Verification items for the finished model (mm, model axes). A direction names the side the tool comes from. Round coordinates to 2 decimals unless told otherwise and drop trailing zeros. Loops run counter-clockwise (first coordinate to the right, second up) from the corner with the lowest first, then second, coordinate; pieces in that order, holes last. Notation, with made-up numbers: M 77.25,24.5 L 123.25,24.5 A13 cw 123.25,47.5 Z; hole C 32.25,19 d2. An arc over 180 degrees is marked long. One line per item, written item: value.
from build123d import *

# Parameters (mm, degrees)
SKETCH_1_W          = 20
SKETCH_1_H          = 20
EXTRUDE_1_DEPTH     = 490
SKETCH_2_W          = 14
SKETCH_2_H          = 14
CUT_EXTRUDE_1_DEPTH = 491
SKETCH_3_R          = 1.5
CUT_EXTRUDE_2_DEPTH = 80
SKETCH_4_R          = 1.55
CUT_EXTRUDE_3_DEPTH = 27


with BuildPart() as part:
    # 草图1 → 凸台-拉伸1 (new body)
    with BuildSketch(Plane.XY):
        with Locations((0.666666667, 1.006147649)):
            Rectangle(SKETCH_1_W, SKETCH_1_H)
    extrude(amount=EXTRUDE_1_DEPTH)

    # 草图2 → 切除-拉伸1 (cut, through all)
    with BuildSketch(Plane(origin=(0, 0, 0), x_dir=(-1, 0, 0), z_dir=(0, 0, -1))):
        with Locations((-0.666666667, 1.006147649)):
            Rectangle(SKETCH_2_W, SKETCH_2_H)
    extrude(amount=-CUT_EXTRUDE_1_DEPTH, mode=Mode.SUBTRACT)

    # 草图3 → 切除-拉伸2 (cut)
    with BuildSketch(Plane(origin=(10.666666667, 0, 0), x_dir=(0, 0, -1), z_dir=(1, 0, 0))):
        with Locations((-477, 1.006147649)):
            Circle(SKETCH_3_R)
        with Locations((-457, 1.006147649)):
            Circle(SKETCH_3_R)
        with Locations((-437, 1.006147649)):
            Circle(SKETCH_3_R)
    extrude(amount=-CUT_EXTRUDE_2_DEPTH, mode=Mode.SUBTRACT)

    # 草图4 → 切除-拉伸3 (cut)
    with BuildSketch(Plane.ZY.offset(9.333333333)):
        with Locations((13, 1.006147649)):
            Circle(SKETCH_4_R)
        with Locations((33, 1.006147649)):
            Circle(SKETCH_4_R)
        with Locations((53, 1.006147649)):
            Circle(SKETCH_4_R)
    extrude(amount=-CUT_EXTRUDE_3_DEPTH, mode=Mode.SUBTRACT)


solid = part.part
(1) Depth check by flat-ended pin: pin 1 Ø2.5 at (y, z) = (1.01, 457) entering from -X. Enter the tip coordinate at first touch or a pass-through.
Completed:
pin 1: passes through
(2) Sectioned sample at A-A on z = 424.5. Enter the section's corners in (x, y), and give its area (3 significant figures).
Completed:
outline: M -9.33,-8.99 L 10.67,-8.99 L 10.67,11.01 L -9.33,11.01 Z; hole M -6.33,-5.99 L 7.67,-5.99 L 7.67,8.01 L -6.33,8.01 Z
area: 204 mm^2
(3) Thickness scan on L1, parallel to X at y = 7.5, z = 412; L2, parallel to Y at x = 0.75, z = 87; L3, parallel to Y at x = 9.65, z = 13. Record the ranges inside material, lowest first. Write a range as from..to.
Completed:
L1: x = -9.33..-6.33, 7.67..10.67
L2: y = -8.99..-5.99, 8.01..11.01
L3: y = -8.99..-0.54, 2.56..11.01
(4) Tool access check on faces 4 (the face through (-8, 1, 490)), 5 (the face through (-6.333, 1, 242)). Record the directions out of +Z, -Z, +X, -X, +Y, -Y that give a thin tool (end or side, any length) a straight path to the whole face; none if there is none.
Completed:
face 4: +Z, +X, -X, +Y, -Y
face 5: +Z, -Z
(5) Mould release check, pull along Y, two halves, no side actions. Record for faces 1 (the face through (1, -8.994, 242)), 2 (the face through (1, 8.006, 242)), 3 (the face through (-8, 1, 0)): +Y half, -Y half, draft (parallel to the pull), parting line (faces both ways), or undercut.
Completed:
face 1: -Y half
face 2: undercut
face 3: draft
(6) Sectioned sample at B-B on x = -3. Enter the section's corners in (y, z), and give its area (3 significant figures).
Completed:
outline: M -8.99,0 L -5.99,0 L -5.99,490 L -8.99,490 Z; M 8.01,0 L 11.01,0 L 11.01,490 L 8.01,490 Z
area: 2,940 mm^2
